```python
from build123d import *

# Parameters (mm, degrees)
SKETCH1_W               = 80
SKETCH1_H               = 80
SKETCH1_R               = 18.4
BOSS_EXTRUDE1_DEPTH     = 2
SKETCH2_W               = 4
SKETCH2_H               = 18.5
BOSS_EXTRUDE2_DEPTH     = 15.25
SKETCH3_R               = 2.2
CUT_EXTRUDE1_DEPTH      = 94.976393312
MIRROR2_COPY_1_SKETCH_W = 4
MIRROR2_COPY_1_SKETCH_H = 18.5
MIRROR2_COPY_1_DEPTH    = 15.25
MIRROR2_COPY_2_SKETCH_R = 2.2
MIRROR2_COPY_2_DEPTH    = 94.976393312
SKETCH4_R               = 2.2
CUT_EXTRUDE2_DEPTH      = 62.388618652
SKETCH5_W               = 4
SKETCH5_H               = 15.25
CUT_EXTRUDE3_DEPTH      = 93.258129723
SKETCH6_W               = 80
SKETCH6_H               = 80
SKETCH6_W_2             = 76
SKETCH6_H_2             = 76
BOSS_EXTRUDE3_DEPTH     = 76


with BuildPart() as part:
    # Sketch1 → Boss-Extrude1 (new body)
    with BuildSketch(Plane(origin=(0, 0, 0), x_dir=(1, 0, 0), z_dir=(0, 1, 0))):
        Rectangle(SKETCH1_W, SKETCH1_H)
        with Locations(Location((0, 0, 0), (0, 0, 270))):
            Circle(SKETCH1_R, mode=Mode.SUBTRACT)
    extrude(amount=BOSS_EXTRUDE1_DEPTH)

    # Sketch2 → Boss-Extrude2 (add)
    with BuildSketch(Plane(origin=(0, 2, 0), x_dir=(1, 0, 0), z_dir=(0, 1, 0))):
        with Locations((42, -30.75)):
            Rectangle(SKETCH2_W, SKETCH2_H)
    boss_extrude2 = extrude(amount=-BOSS_EXTRUDE2_DEPTH)

    # Sketch3 → Cut-Extrude1 (cut, through all)
    with BuildSketch(Plane(origin=(44, 0, 0), x_dir=(0, 0, -1), z_dir=(1, 0, 0))):
        with Locations((-30.75, -8.125)):
            Circle(SKETCH3_R)
    cut_extrude1 = extrude(amount=-CUT_EXTRUDE1_DEPTH, mode=Mode.SUBTRACT)

    # Mirror1: Boss-Extrude2, Cut-Extrude1 across plane
    add(boss_extrude2.mirror(Plane(origin=(0, 0, 0), x_dir=(0, 0, 1), z_dir=(1, 0, 0))))
    add(cut_extrude1.mirror(Plane(origin=(0, 0, 0), x_dir=(0, 0, 1), z_dir=(1, 0, 0))), mode=Mode.SUBTRACT)

    # Mirror2: Boss-Extrude2, Cut-Extrude1 across plane
    add(boss_extrude2.mirror(Plane(origin=(0, 0, 0), x_dir=(1, 0, 0), z_dir=(0, 0, -1))))
    add(cut_extrude1.mirror(Plane(origin=(0, 0, 0), x_dir=(1, 0, 0), z_dir=(0, 0, -1))), mode=Mode.SUBTRACT)

    # Mirror2 copy 1 sketch → Mirror2 copy 1 (add)
    with BuildSketch(Plane(origin=(0, 2, 0), x_dir=(-1, 0, 0), z_dir=(0, 1, 0))):
        with Locations((42, -30.75)):
            Rectangle(MIRROR2_COPY_1_SKETCH_W, MIRROR2_COPY_1_SKETCH_H)
    extrude(amount=-MIRROR2_COPY_1_DEPTH)

    # Mirror2 copy 2 sketch → Mirror2 copy 2 (cut, through all)
    with BuildSketch(Plane.ZY.offset(44)):
        with Locations((-30.75, -8.125)):
            Circle(MIRROR2_COPY_2_SKETCH_R)
    extrude(amount=-MIRROR2_COPY_2_DEPTH, mode=Mode.SUBTRACT)

    # Sketch4 → Cut-Extrude2 (cut, through all)
    with BuildSketch(Plane(origin=(0, 2, 0), x_dir=(1, 0, 0), z_dir=(0, 1, 0))):
        with Locations(Location((-24, 24, 0), (0, 0, 270))):
            Circle(SKETCH4_R)
        with Locations(Location((24, 24, 0), (0, 0, 270))):
            Circle(SKETCH4_R)
    cut_extrude2 = extrude(amount=-CUT_EXTRUDE2_DEPTH, mode=Mode.SUBTRACT)

    # Mirror3: Cut-Extrude2 across plane
    add(cut_extrude2.mirror(Plane(origin=(0, 0, 0), x_dir=(1, 0, 0), z_dir=(0, 0, -1))), mode=Mode.SUBTRACT)

    # Sketch5 → Cut-Extrude3 (cut, through all)
    with BuildSketch(Plane.XY.offset(40)):
        with Locations((-42, -5.625)):
            Rectangle(SKETCH5_W, SKETCH5_H)
        with Locations((42, -5.625)):
            Rectangle(SKETCH5_W, SKETCH5_H)
    extrude(amount=-CUT_EXTRUDE3_DEPTH, mode=Mode.SUBTRACT)

    # Sketch6 → Boss-Extrude3 (add)
    with BuildSketch(Plane(origin=(0, 2, 0), x_dir=(1, 0, 0), z_dir=(0, 1, 0))):
        Rectangle(SKETCH6_W, SKETCH6_H)
        Rectangle(SKETCH6_W_2, SKETCH6_H_2, mode=Mode.SUBTRACT)
    extrude(amount=BOSS_EXTRUDE3_DEPTH)


solid = part.part
```
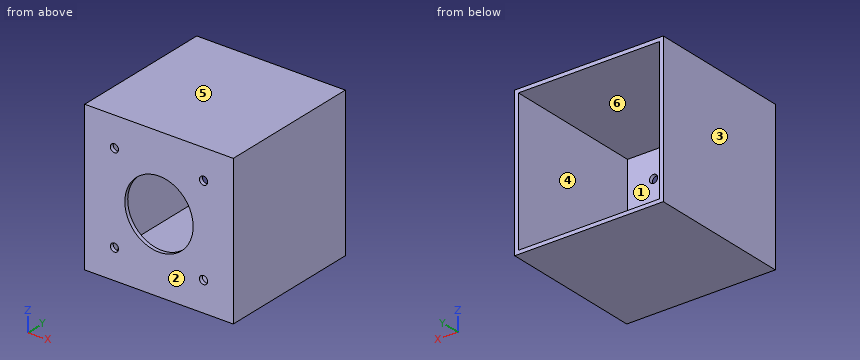
Verification items for the finished model (mm, model axes). Face numbers are marked on the shaded views. A direction names the side the tool comes from. Coordinates: 2 decimals unless noted, no trailing zeros. Order: outer loops, then holes, each group sorted by start corner. A loop starts at its lowest first (then second) coordinate and runs counter-clockwise, first axis right, second up. Notation, with made-up numbers: (31.25, 26.5) -> (78.25, 26.5) arc R18 cw to (78.25, 35.5) -> close; hole circle Ø2 at (64, 17.5). An arc over 180 degrees is marked (long way). Answer as CSV lines item,"result". Start each with the question number.
1) Cross-section at A-A, the plane x = -24. Record the boundary of the cut face in (y, z), then the cut area to 3 significant figures.
2) Set-up check for the marked faces 1 and 2: record each of +Z, -Z, +X, -X, +Y, -Y from which the full face is reachable in a straight line by a thin tool's end or side.
3) Cross-section at B-B, the plane y = 59. Record the boundary of the cut face in (x, z), then the cut area to 3 significant figures.
4) Cross-section at C-C, the plane x = 0. Record the boundary of the cut face in (y, z).
5) Release check for a two-part mould opening along Z. For the marked faces 3, 4, 5 and 6 record: released by +Z, released by -Z, zero draft, split by the parting line, or undercut.
6) Material ranges on L1, parallel to X at y = 1.3, z = 24; L2, parallel to Z at x = 3, y = 42.5, recorded low to high. Write a range as [from, to].
7) Cross-section at D-D, the plane z = 24. Record the boundary of the cut face in (x, y), then the cut area to 3 significant figures.
8) Gauge pin test, flat ends, axial feed: pin 1 Ø23 at (x, z) = (18, 9.5) entering from +Y; pin 2 Ø2.5 at (x, z) = (-24, -24) entering from -Y. Record the tip position at first contact, or that the pin passes through.
Conclusion:
1,outline,"(0, -40) -> (78, -40) -> (78, -38) -> (2, -38) -> (2, -26.2) -> (0, -26.2) -> close; (0, -21.8) -> (2, -21.8) -> (2, 21.8) -> (0, 21.8) -> close; (0, 26.2) -> (2, 26.2) -> (2, 38) -> (78, 38) -> (78, 40) -> (0, 40) -> close"
1,area,"446 mm²"
2,face 1,"+Y"
2,face 2,"+Z, -Z, +X, -X, -Y"
3,outline,"(-40, -40) -> (40, -40) -> (40, 40) -> (-40, 40) -> close; hole (-38, -38) -> (38, -38) -> (38, 38) -> (-38, 38) -> close"
3,area,"624 mm²"
4,outline,"(0, -40) -> (78, -40) -> (78, -38) -> (2, -38) -> (2, -18.4) -> (0, -18.4) -> close; (0, 18.4) -> (2, 18.4) -> (2, 38) -> (78, 38) -> (78, 40) -> (0, 40) -> close"
5,face 3,"zero draft"
5,face 4,"undercut"
5,face 5,"released by +Z"
5,face 6,"undercut"
6,L1,"x = [-40, -26.2], [-21.8, 21.8], [26.2, 40]"
6,L2,"z = [-40, -38], [38, 40]"
7,outline,"(-40, 0) -> (-26.2, 0) -> (-26.2, 2) -> (-38, 2) -> (-38, 78) -> (-40, 78) -> close; (-21.8, 0) -> (21.8, 0) -> (21.8, 2) -> (-21.8, 2) -> close; (26.2, 0) -> (40, 0) -> (40, 78) -> (38, 78) -> (38, 2) -> (26.2, 2) -> close"
7,area,"446 mm²"
8,pin 1,"stops at y = 2"
8,pin 2,"passes through"
